The listing builds one solid part. Answer for the finished solid, in the listing's coordinates (mm). A direction names the side the tool comes from. Give positions to 0.01 mm unless a question says otherwise; leave off trailing zeros. Write each loop counter-clockwise with the first axis right and the second up, starting at its lowest first coordinate (ties: lowest second). Pieces come first, ordered by that corner, then holes. Notation, with made-up numbers: (81, -33.5) - (88, -33.5) arc R15 cw to (88, -27.5) - close; hole circle Ø6 at (62.25, -15.5). An arc over 180 degrees is marked (long way). Return JSON: item names as keys, results as strings.
from build123d import *

# Parameters (mm, degrees)
SKETCH1_R           = 12.5
BOSS_EXTRUDE1_DEPTH = 250
CHAMFER1_SIZE       = 2
CUT_EXTRUDE1_START  = -20
SKETCH3_R           = 12.5
SKETCH3_R_2         = 10
CUT_EXTRUDE1_DEPTH  = 20


with BuildPart() as part:
    # Sketch1 → Boss-Extrude1 (new, symmetric)
    with BuildSketch(Plane(origin=(0, 0, 0), x_dir=(1, 0, 0), z_dir=(0, 1, 0))):
        with Locations(Location((0, 0, 0), (0, 0, 270))):
            Circle(SKETCH1_R)
    extrude(amount=BOSS_EXTRUDE1_DEPTH, both=True)

    # Chamfer1
    chamfer1_edges = [part.edges().sort_by_distance(p)[0] for p in [
        (0, 250, -12.5),
    ]]
    chamfer(chamfer1_edges, length=CHAMFER1_SIZE)

    # Sketch3 → Cut-Extrude1 (cut)
    with BuildSketch(Plane.XZ.offset(250).offset(CUT_EXTRUDE1_START)):
        with Locations(Location((0, 0, 0), (0, 0, 270))):
            Circle(SKETCH3_R)
        with Locations(Location((0, 0, 0), (0, 0, 270))):
            Circle(SKETCH3_R_2, mode=Mode.SUBTRACT)
    extrude(amount=CUT_EXTRUDE1_DEPTH, mode=Mode.SUBTRACT)


solid = part.part
Item 1: Flat-ended cylindrical pins translate along their axes: P1, Ø2, axis at x = 2, y = 168, coming from the +Z side; P2, Ø5, axis at x = -4, y = -109, coming from the -Z side; P3, Ø8, axis at y = -32.5, z = 6, coming from the +X side. Find the tip coordinate at first contact, or state that the pin passes through.
Answer below:
{"P1": "stops at z = 12.46", "P2": "stops at z = -12.41", "P3": "stops at x = 12.34"}
Item 2: A cutting plane is placed at A-A on y = -134.5. Determine the outline of the cut face in (x, z), then the cut area to 3 significant figures.
Answer below:
{"outline": "circle Ø25 at (0, 0)", "area": "491 mm²"}
Item 3: Consider L1, parallel to X at y = 110.5, z = -6.75; L2, parallel to Z at x = 0.5, y = 108.5; L3, parallel to X at y = -34, z = -0.75. Determine where each line is inside the solid, lowest interval first.
Answer below:
{"L1": "x = -10.52 to 10.52", "L2": "z = -12.49 to 12.49", "L3": "x = -12.48 to 12.48"}
Item 4: For faces 1 (the face through (0, -250, 0)), 2 (the face through (10.2, -230, 0.1)), determine the directions among +Z, -Z, +X, -X, +Y, -Y from which every point of the face is accessible in a straight line to the end or side of a thin tool.
Answer below:
{"face 1": "+Z, -Z, +X, -X, -Y", "face 2": "-Y"}
